Part model, mm, in its own coordinate system. A direction names the side the tool comes from. Round coordinates to 2 decimals unless told otherwise and drop trailing zeros. Loops run counter-clockwise (first coordinate to the right, second up) from the corner with the lowest first, then second, coordinate; pieces in that order, holes last. Notation, with made-up numbers: (-12.75, 65) -> (8.25, 65) arc R11 ccw to (8.25, 86) -> close; hole circle Ø4 at (-3, 74.5). An arc over 180 degrees is marked (long way). Use a Markdown table: item, result. Add a question column.
Item 1: Two-plate mould, pull along X, no slides. Class faces 5 (the face through (-27.1, 64.14, 2.54)), 6 (the face through (-7.7, 35.1, 0)), 7 (the face through (-24, 7, 3)): pulls with the +X half, pulls with the -X half, needs draft (parallel to the pull), parting line crosses it, or undercut.
Item 2: Which spindle directions (+Z, -Z, +X, -X, +Y, -Y) get a long thin tool onto all of the face, cutting with end or side? Do faces 1 (the face through (-23.6, 7, 3)), 2 (the face through (-16, 0, 2)), 3 (the face through (-24, 57, 2)), 4 (the face through (11, 57, 2)). Say none if no direction does.
Item 3: Cut at C-C, the plane z = 1.3. List the corners of the cut face in (x, y), plus the area to 3 significant figures.
Item 4: Cut at B-B, the plane y = 58. List the corners of the cut face in (x, z).
Item 5: Cut at D-D, the plane y = 28. List the corners of the cut face in (x, z).
Item 6: Flat gauge pins, fed straight in: pin 1 (0.9 mm diameter, centred on y = 6.5, z = 3, fed in from +X); pin 2 (1.5 mm diameter, centred on y = 59, z = 2.5, fed in from +X); pin 3 (4 mm diameter, centred on x = 0.5, y = 23, fed in from +Z); pin 4 (3 mm diameter, centred on x = 4, z = 4, fed in from -Y). Where does each tip first touch, or does it go through?
Item 7: Probe line 1 (Y direction, x = -22.5, z = 2.4); line 2 (Y direction, x = 8.5, z = 2.05); line 3 (X direction, y = 45, z = 2.6). List the from-to ranges inside material, lowest first. Write a range as [from, to].
Item 8: Cut at A-A, the plane x = -20. List the corners of the cut face in (y, z), plus the area to 3 significant figures.
```python
from build123d import *

# Parameters (mm, degrees)
BOSS_EXTRUDE1_DEPTH = 5
SKETCH2_W           = 0.4
SKETCH2_H           = 5
CUT_EXTRUDE1_DEPTH  = 3
SKETCH3_W           = 0.1
SKETCH3_H           = 5
CUT_EXTRUDE2_DEPTH  = 3
FILLET1_R           = 5
FILLET2_R           = 3
FILLET3_R           = 1


with BuildPart() as part:
    # Sketch1 → Boss-Extrude1 (new body)
    with BuildSketch(Plane.XY):
        Polygon((0, 65), (-28, 65), (-28, 57), (-8, 57), (-8, 8), (-28, 8), (-28, 0), (0, 0), (0, 57), (20, 57), (20, 65), align=None)
    extrude(amount=BOSS_EXTRUDE1_DEPTH)

    # Sketch2 → Cut-Extrude1 (cut)
    with BuildSketch(Plane(origin=(0, 8, 0), x_dir=(1, 0, 0), z_dir=(0, 1, 0))):
        with Locations((-23.8, -2.5)):
            Rectangle(SKETCH2_W, SKETCH2_H)
    extrude(amount=-CUT_EXTRUDE1_DEPTH, mode=Mode.SUBTRACT)

    # Sketch3 → Cut-Extrude2 (cut)
    with BuildSketch(Plane.XZ.offset(-57)):
        with Locations((-23.6, 2.5)):
            Rectangle(SKETCH3_W, SKETCH3_H)
    extrude(amount=-CUT_EXTRUDE2_DEPTH, mode=Mode.SUBTRACT)

    # Fillet1
    fillet1_edges = [part.edges().sort_by_distance(p)[0] for p in [
        (0, 0, 2.5),
        (-8, 8, 2.5),
        (-8, 57, 2.5),
        (0, 57, 2.5),
    ]]
    fillet(fillet1_edges, radius=FILLET1_R)

    # Fillet2
    fillet2_edges = [part.edges().sort_by_distance(p)[0] for p in [
        (-28, 57, 2.5),
        (-28, 65, 2.5),
        (20, 65, 2.5),
        (20, 57, 2.5),
    ]]
    fillet(fillet2_edges, radius=FILLET2_R)

    # Fillet3
    fillet3_edges = [part.edges().sort_by_distance(p)[0] for p in [
        (-28, 0, 2.5),
        (-28, 8, 2.5),
    ]]
    fillet(fillet3_edges, radius=FILLET3_R)


solid = part.part
```
A:
| question | item | result |
|---|---|---|
| 1 | face 5 | pulls with the -X half |
| 1 | face 6 | needs draft |
| 1 | face 7 | undercut |
| 2 | face 1 | +Z, -Z |
| 2 | face 2 | +Z, -Z, +X, -X, -Y |
| 2 | face 3 | +Z, -Z, -X |
| 2 | face 4 | +Z, -Z, +X, -Y |
| 3 | outline | (-28, 1) arc R1 ccw to (-27, 0) -> (-5, 0) arc R5 ccw to (0, 5) -> (0, 52) arc R5 cw to (5, 57) -> (17, 57) arc R3 ccw to (20, 60) -> (20, 62) arc R3 ccw to (17, 65) -> (-25, 65) arc R3 ccw to (-28, 62) -> (-28, 60) arc R3 ccw to (-25, 57) -> (-23.65, 57) -> (-23.65, 60) -> (-23.55, 60) -> (-23.55, 57) -> (-13, 57) arc R5 cw to (-8, 52) -> (-8, 13) arc R5 cw to (-13, 8) -> (-23.6, 8) -> (-23.6, 5) -> (-24, 5) -> (-24, 8) -> (-27, 8) arc R1 ccw to (-28, 7) -> close |
| 3 | area | 1,000 mm^2 |
| 4 | outline | (-27.24, 0) -> (-23.65, 0) -> (-23.65, 5) -> (-27.24, 5) -> close; (-23.55, 0) -> (19.24, 0) -> (19.24, 5) -> (-23.55, 5) -> close |
| 5 | outline | (-8, 0) -> (0, 0) -> (0, 5) -> (-8, 5) -> close |
| 6 | pin 1 | stops at x = 0 |
| 6 | pin 2 | stops at x = 19.99 |
| 6 | pin 3 | stops at z = 5 |
| 6 | pin 4 | stops at y = 56.33 |
| 7 | line 1 | y = [0, 8], [57, 65] |
| 7 | line 2 | y = [57, 65] |
| 7 | line 3 | x = [-8, 0] |
| 8 | outline | (0, 0) -> (8, 0) -> (8, 5) -> (0, 5) -> close; (57, 0) -> (65, 0) -> (65, 5) -> (57, 5) -> close |
| 8 | area | 80.0 mm^2 |
